The listing builds one solid part. Answer for the finished solid, in the listing's coordinates (mm). Face numbers are marked on the shaded views. A direction names the side the tool comes from. Round coordinates to 2 decimals unless told otherwise and drop trailing zeros. Loops run counter-clockwise (first coordinate to the right, second up) from the corner with the lowest first, then second, coordinate; pieces in that order, holes last. Notation, with made-up numbers: (53, 17.5) -> (94, 17.5) arc R18 ccw to (94, 46.5) -> close; hole circle Ø9 at (43, -7). An arc over 180 degrees is marked (long way). Write each question's results on one line, items separated by ' | '. Start each with the question number.
(1) Determine the mould class of the marked faces 1, 2, 3 and 4 for opening direction Y: released by +Y, released by -Y, zero draft, split by the parting line, or undercut.
(2) The part is cut by section C-C (z = 7.25). Determine the outline of the cut face in (x, y), plus the area to 3 significant figures.
(3) The part is cut by section B-B (x = -2.75). Determine the outline of the cut face in (y, z), plus the area to 3 significant figures.
(4) The part is cut by section A-A (y = 2.5). Determine the outline of the cut face in (x, z), plus the area to 3 significant figures.
(5) For the marked faces 5 and 6, determine the directions among +Z, -Z, +X, -X, +Y, -Y from which every point of the face is accessible in a straight line to the end or side of a thin tool.
(6) The part is cut by section D-D (y = 5.75). Determine the outline of the cut face in (x, z), plus the area to 3 significant figures.
(7) Straight lines are drawn through the part: probe 1 along Y at (x, z) = (1.75, 12.25); probe 2 along X at (y, z) = (1.75, 16.5); probe 3 along Z at (x, y) = (-4.5, -1.25). For each, find the intervals that lie inside material, in ascending order.
(8) Flat-ended cylindrical pins translate along their axes: pin 1 (1.6 mm diameter, centred on x = -8.5, y = -0.5, fed in from -Z); pin 2 (1.2 mm diameter, centred on y = -9.5, z = 1, fed in from -X); pin 3 (1.2 mm diameter, centred on x = -8.5, y = -1, fed in from +Z); pin 4 (0.8 mm diameter, centred on x = -8.5, z = 2.5, fed in from +Y). Find the tip coordinate at first contact, or state that the pin passes through.
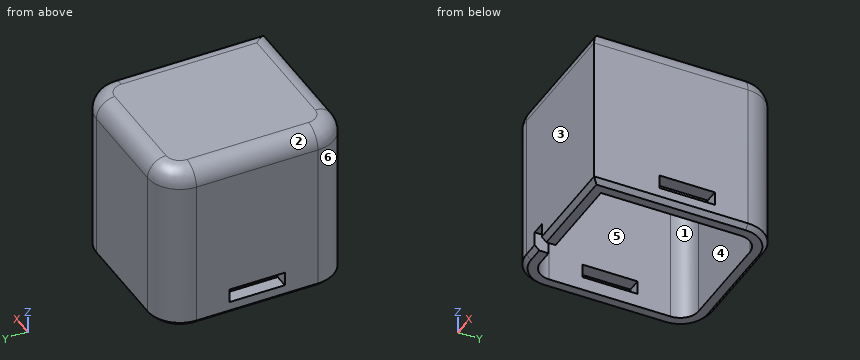
Autodesk Inventor part; units mm, degrees
ref_plane "YZ Plane" through (0, 0, 0) normal (1, 0, 0) x (0, 1, 0)
ref_plane "XZ Plane" through (0, 0, 0) normal (0, 1, 0) x (-1, 0, 0)
ref_plane "XY Plane" through (0, 0, 0) normal (0, 0, 1) x (1, 0, 0)
sketch "스케치1" plane through (0, 0, 0) normal (0, 0, 1) x (1, 0, 0)
  line L0 (-5.4, -8.6) -> (7.4, -8.6)
  line L1 (7.4, -8.6) -> (7.4, 6.6)
  line L2 (5.4, 8.6) -> (-5.4, 8.6)
  line L3 (-7.4, 6.6) -> (-7.4, -6.6)
  line L4 (-7.4, -8.6) -> (7.4, 8.6) construction
  line L5 (7.4, -8.6) -> (-7.4, 8.6) construction
  arc A0 (-5.4, 8.6) -> (-7.4, 6.6) centre (-5.4, 6.6) ccw
  arc A1 (7.4, 6.6) -> (5.4, 8.6) centre (5.4, 6.6) ccw
  arc A2 (-7.4, -6.6) -> (-5.4, -8.6) centre (-5.4, -6.6) ccw
  line L6 (-5.4, 10.1) -> (5.4, 10.1)
  arc A3 (8.9, 6.6) -> (5.4, 10.1) centre (5.4, 6.6) ccw
  line L7 (8.9, 6.6) -> (8.9, -10.1)
  line L8 (8.9, -10.1) -> (-5.4, -10.1)
  arc A4 (-8.9, -6.6) -> (-5.4, -10.1) centre (-5.4, -6.6) ccw
  line L9 (-8.9, -6.6) -> (-8.9, 6.6)
  arc A5 (-5.4, 10.1) -> (-8.9, 6.6) centre (-5.4, 6.6) ccw
  point P0 (0, 0)
  dimension "d0" = 17.2
  dimension "d1" = 14.8
  dimension "d2" = 2
  dimension "d3" = 1.5
extrude "돌출1" add sketch "스케치1" along normal blind 17
sketch "스케치2" plane through (0, 0, 17) normal (0, 0, 1) x (1, 0, 0)
  line L0 (-5.4, -10.1) -> (8.9, -10.1)
  line L1 (8.9, -10.1) -> (8.9, 6.6)
  arc A0 (8.9, 6.6) -> (5.4, 10.1) centre (5.4, 6.6) ccw
  line L2 (5.4, 10.1) -> (-5.4, 10.1)
  arc A1 (-5.4, 10.1) -> (-8.9, 6.6) centre (-5.4, 6.6) ccw
  line L3 (-8.9, 6.6) -> (-8.9, -6.6)
  arc A2 (-8.9, -6.6) -> (-5.4, -10.1) centre (-5.4, -6.6) ccw
  point P0 (0, 0)
extrude "돌출2" add sketch "스케치2" along normal blind 1.5
sketch "스케치3" plane through (-8.9, -6.6, 0) normal (-1, 0, 0) x (0, 0, 1)
  line L0 (0, 13.2) -> (0, 0)
  line L1 (3, 3.6) -> (1.5, 3.6)
  line L2 (1.5, 3.6) -> (1.5, 9.6)
  line L3 (1.5, 9.6) -> (3, 9.6)
  line L4 (3, 9.6) -> (3, 3.6)
  point P0 (0, 6.6)
  point P1 (0, 6.6)
  point P2 (1.5, 6.6)
  dimension "d8" = 6
  dimension "d9" = 1.5
  dimension "d10" = 1.5
extrude "돌출3" cut sketch "스케치3" against normal through all
fillet "모깎기1" radius 2 7 edges at (-7.8749, -9.0749, 18.5) (1.75, -10.1, 18.5) (-7.8749, 9.0749, 18.5) (0, 10.1, 18.5) (7.8749, 9.0749, 18.5) (8.9, -1.75, 18.5) (-8.9, 0, 18.5)
chamfer "모따기1" distance 0.5 angle 45 7 edges at (1.75, -10.1, 0) (-7.8749, -9.0749, 0) (-8.9, 0, 0) (-7.8749, 9.0749, 0) (0, 10.1, 0) (7.8749, 9.0749, 0) (8.9, -1.75, 0)
sketch "스케치4" plane through (-5.4, -10.1, 16.5) normal (0, -1, 0) x (1, 0, 0)
  line L0 (1.75, -14.5) -> (3.25, -14.5)
  line L1 (3.25, -14.5) -> (3.25, -16.5)
  line L2 (3.25, -16.5) -> (1.75, -16.5)
  line L3 (1.75, -16.5) -> (1.75, -14.5)
  line L4 (-3.5, -16) -> (-3.5, 0)
  line L5 (0, -16.5) -> (13.8, -16.5)
  point P0 (5.4, -16.5)
  point P1 (2.5, -14.5)
  point P2 (2.5, -14.5)
  dimension "d17" = 1.5
  dimension "d18" = 2
  dimension "d19" = 6
extrude "돌출4" cut sketch "스케치4" against normal up to surface (1.5 mm away)
properties part number "_3D 인쇄"
Checked values:
1) face 1: undercut | face 2: zero draft | face 3: released by -Y | face 4: undercut
2) outline: (-8.9, -6.6) arc R3.5 ccw to (-5.4, -10.1) -> (8.9, -10.1) -> (8.9, 6.6) arc R3.5 ccw to (5.4, 10.1) -> (-5.4, 10.1) arc R3.5 ccw to (-8.9, 6.6) -> close; hole (-7.4, -6.6) arc R2 ccw to (-5.4, -8.6) -> (7.4, -8.6) -> (7.4, 6.6) arc R2 ccw to (5.4, 8.6) -> (-5.4, 8.6) arc R2 ccw to (-7.4, 6.6) -> close | area: 99.7 mm2
3) outline: (-10.1, 2) -> (-8.6, 2) -> (-8.6, 17) -> (8.6, 17) -> (8.6, 0) -> (9.6, 0) -> (10.1, 0.5) -> (10.1, 16.5) arc R2 ccw to (8.1, 18.5) -> (-8.1, 18.5) arc R2 ccw to (-10.1, 16.5) -> close | area: 76.5 mm2
4) outline: (-8.9, 0.5) -> (-8.4, 0) -> (-7.4, 0) -> (-7.4, 1.5) -> (-8.9, 1.5) -> close; (-8.9, 3) -> (-7.4, 3) -> (-7.4, 17) -> (7.4, 17) -> (7.4, 3) -> (8.9, 3) -> (8.9, 16.5) arc R2 ccw to (6.9, 18.5) -> (-6.9, 18.5) arc R2 ccw to (-8.9, 16.5) -> close; (7.4, 0) -> (8.4, 0) -> (8.9, 0.5) -> (8.9, 1.5) -> (7.4, 1.5) -> close | area: 71.2 mm2
5) face 5: -Z | face 6: +Z, -Z, -X, -Y
6) outline: (-8.9, 0.5) -> (-8.4, 0) -> (-7.4, 0) -> (-7.4, 17) -> (7.4, 17) -> (7.4, 0) -> (8.4, 0) -> (8.9, 0.5) -> (8.9, 16.5) arc R2 ccw to (6.9, 18.5) -> (-6.9, 18.5) arc R2 ccw to (-8.9, 16.5) -> close | area: 75.7 mm2
7) probe 1: y = -10.1 to -8.6, 8.6 to 10.1 | probe 2: x = -8.9 to -7.4, 7.4 to 8.9 | probe 3: z = 17 to 18.5
8) pin 1: stops at z = 0 | pin 2: stops at x = -8.04 | pin 3: stops at z = 18.23 | pin 4: stops at y = 8.83
